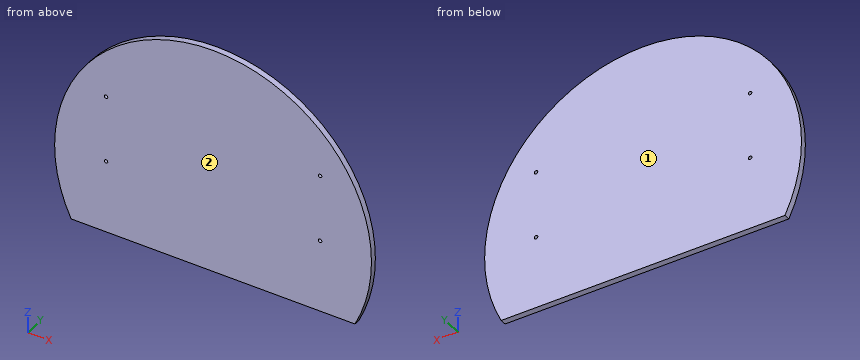
from build123d import *

# Parameters (mm, degrees)
SKETCH1_R             = 164.975
BOSS_EXTRUDE1_DEPTH   = 6.35
F_6_CLEARANCE_HOLE1_D = 3.6576
CUT_EXTRUDE1_START    = -6.35
CUT_EXTRUDE1_DEPTH    = 6.35


with BuildPart() as part:
    # Sketch1 → Boss-Extrude1 (new body)
    with BuildSketch(Plane(origin=(0, 0, 0), x_dir=(1, 0, 0), z_dir=(0, 1, 0))):
        with Locations(Location((0, 0, 0), (0, 0, 270))):
            Circle(SKETCH1_R)
    extrude(amount=BOSS_EXTRUDE1_DEPTH)

    # #6 Clearance Hole1 (through all)
    with Locations(Plane(origin=(111.465, 0, 2.54), x_dir=(0, 0, -1), z_dir=(0, -1, 0))):
        with Locations((0, 0), (-69.85, 0), (-69.85, -222.93), (0, -222.93)):
            Hole(F_6_CLEARANCE_HOLE1_D / 2)

    # Sketch9 → Cut-Extrude1 (cut)
    with BuildSketch(Plane(origin=(0, 6.35, 0), x_dir=(1, 0, 0), z_dir=(0, 1, 0)).offset(CUT_EXTRUDE1_START)):
        with BuildLine():
            Line((-147.793016902, 73.307399216), (147.793016902, 73.307399216))
            ThreePointArc((147.793016902, 73.307399216), (0, 164.975), (-147.793016902, 73.307399216))
        make_face()
    extrude(amount=CUT_EXTRUDE1_DEPTH, mode=Mode.SUBTRACT)


solid = part.part
Source: CAD feature listing. Evaluate the final solid. Frame: model axes, mm. Face numbers are marked on the shaded views. Coordinates: 2 decimals unless noted, no trailing zeros. Order: outer loops, then holes, each group sorted by start corner. A loop starts at its lowest first (then second) coordinate and runs counter-clockwise, first axis right, second up. Notation, with made-up numbers: M 30,8.25 L 76,8.25 A19 cw 76,43.25 Z; hole C 26.5,79 d1. An arc over 180 degrees is marked long. Write each question's results on one line, items separated by ' | '. Start each with the question number.
1. Pin query (flat end, axial travel): pin 1 (5 mm diameter, centred on x = 111.465, z = 2.54, fed in from +Y); pin 2 (1 mm diameter, centred on x = 19.5, y = 3, fed in from +Z); pin 3 (1.5 mm diameter, centred on y = 4, z = 131, fed in from -X). Return the tip coordinate at first contact, or that it passes through.
2. Material intervals for L1, parallel to X at y = 2.5, z = 2.54; L2, parallel to X at y = 4.75, z = 72.39; L3, parallel to Z at x = -112, y = 3.5, sorted ascending.
3. Section A-A, the plane y = 1.75. Return the cut outline in (x, z) (3 decimals), then the cut area to 3 significant figures.
4. Section B-B, the plane z = 82. Return the cut outline in (x, y).
5. Draft query along Y for the marked faces 1 and 2. Return one class per face: +Y half, -Y half, draft (parallel to the pull), parting line (faces both ways), or undercut.
6. Section C-C, the plane x = -57.5. Return the cut outline in (y, z), then the cut area to 3 significant figures.
Solution:
1) pin 1: y = 6.35 | pin 2: z = 163.88 | pin 3: x = -101.25
2) L1: -164.96 to -113.29, -109.64 to 109.64, 113.29 to 164.96 | L2: -148.24 to -113.29, -109.64 to 109.64, 113.29 to 148.24 | L3: -73.31 to 0.79, 4.29 to 70.64, 74.14 to 121.13
3) outline: M -147.793,-73.307 L 147.793,-73.307 A164.975 ccw long Z; hole C -111.465,2.54 d3.658; hole C -111.465,72.39 d3.658; hole C 111.465,2.54 d3.658; hole C 111.465,72.39 d3.658 | area: 66,100 mm²
4) outline: M -143.15,0 L 143.15,0 L 143.15,6.35 L -143.15,6.35 Z
5) face 1: +Y half | face 2: -Y half
6) outline: M 0,-73.31 L 6.35,-73.31 L 6.35,154.63 L 0,154.63 Z | area: 1,450 mm²
